Here's how the part is built. I have some questions about the finished solid (model axes, mm). Give positions to 0.01 mm unless a question says otherwise; leave off trailing zeros. Loops run counter-clockwise (first coordinate to the right, second up) from the corner with the lowest first, then second, coordinate; pieces in that order, holes last. Notation, with made-up numbers: (72, 57) - (125, 57) arc R26 cw to (125, 94) - close; hole circle Ø6 at (25, -7.5). An arc over 180 degrees is marked (long way). Use a Markdown table: item, result.
from build123d import *

# Parameters (mm, degrees)
SKETCH1_W           = 88.9
SKETCH1_H           = 88.9
BOSS_EXTRUDE1_DEPTH = 2.54
SKETCH2_R           = 3.175
CUT_EXTRUDE1_DEPTH  = 6.08
FILLET1_R           = 5.08


with BuildPart() as part:
    # Sketch1 → Boss-Extrude1 (new body, symmetric)
    with BuildSketch(Plane.XY):
        with Locations((44.45, 44.45)):
            Rectangle(SKETCH1_W, SKETCH1_H)
    extrude(amount=BOSS_EXTRUDE1_DEPTH, both=True)

    # Sketch2 → Cut-Extrude1 (cut, through all)
    with BuildSketch(Plane.XY.offset(2.54)):
        with Locations((6.35, 82.55)):
            Circle(SKETCH2_R)
        with Locations((82.55, 82.55)):
            Circle(SKETCH2_R)
        with Locations((82.55, 6.35)):
            Circle(SKETCH2_R)
        with Locations((6.35, 6.35)):
            Circle(SKETCH2_R)
        with Locations((44.45, 44.45)):
            Circle(SKETCH2_R)
    extrude(amount=-CUT_EXTRUDE1_DEPTH, mode=Mode.SUBTRACT)

    # Fillet1
    fillet1_edges = [part.edges().sort_by_distance(p)[0] for p in [
        (0, 88.9, 0),
        (88.9, 88.9, 0),
        (88.9, 0, 0),
        (0, 0, 0),
    ]]
    fillet(fillet1_edges, radius=FILLET1_R)


solid = part.part
(1) If I drill on line 1 (Y direction, x = 6.35, z = 1.3) (3 decimals); line 2 (X direction, y = 83.5, z = -0.95), over which ranges is the centre line in solid material (lowest first)?
A:
| item | result |
|---|---|
| line 1 | 0 to 3.175, 9.525 to 79.375, 85.725 to 88.9 |
| line 2 | 0 to 3.32, 9.38 to 79.52, 85.58 to 88.9 |
(2) Suppose I cut it at A-A on y = 6.35. Write out the boundary of the cut face in (x, z) (3 decimals).
A:
| item | result |
|---|---|
| outline | (0, -2.54) - (3.175, -2.54) - (3.175, 2.54) - (0, 2.54) - close; (9.525, -2.54) - (79.375, -2.54) - (79.375, 2.54) - (9.525, 2.54) - close; (85.725, -2.54) - (88.9, -2.54) - (88.9, 2.54) - (85.725, 2.54) - close |
(3) Suppose I cut it at B-B on x = 44.45. Write out the boundary of the cut face in (y, z) (3 decimals), plus the area to 3 significant figures.
A:
| item | result |
|---|---|
| outline | (0, -2.54) - (41.275, -2.54) - (41.275, 2.54) - (0, 2.54) - close; (47.625, -2.54) - (88.9, -2.54) - (88.9, 2.54) - (47.625, 2.54) - close |
| area | 419 mm2 |
(4) Suppose I cut it at C-C on z = -1.4. Write out the boundary of the cut face in (x, y) (3 decimals), plus the area to 3 significant figures.
A:
| item | result |
|---|---|
| outline | (0, 5.08) arc R5.08 ccw to (5.08, 0) - (83.82, 0) arc R5.08 ccw to (88.9, 5.08) - (88.9, 83.82) arc R5.08 ccw to (83.82, 88.9) - (5.08, 88.9) arc R5.08 ccw to (0, 83.82) - close; hole circle Ø6.35 at (6.35, 6.35); hole circle Ø6.35 at (6.35, 82.55); hole circle Ø6.35 at (44.45, 44.45); hole circle Ø6.35 at (82.55, 6.35); hole circle Ø6.35 at (82.55, 82.55) |
| area | 7,720 mm2 |
(5) Will these pins go through, and if not, where does the flat tip stop? pin 1 (5.5 mm diameter, centred on x = 6.35, y = 6.35, fed in from +Z); pin 2 (10 mm diameter, centred on x = 82.55, y = 82.55, fed in from +Z).
A:
| item | result |
|---|---|
| pin 1 | through |
| pin 2 | z = 2.54 |
(6) We'd pull the mould along Y, two halves only. Please class faces 1 (the face through (44, 88.9, 0)), 2 (the face through (42.11, 46.596, 0.036)), 3 (the face through (88.9, 44, 0)): pulls with the +Y half, pulls with the -Y half, needs draft (parallel to the pull), parting line crosses it, or undercut.
A:
| item | result |
|---|---|
| face 1 | pulls with the +Y half |
| face 2 | undercut |
| face 3 | needs draft |
